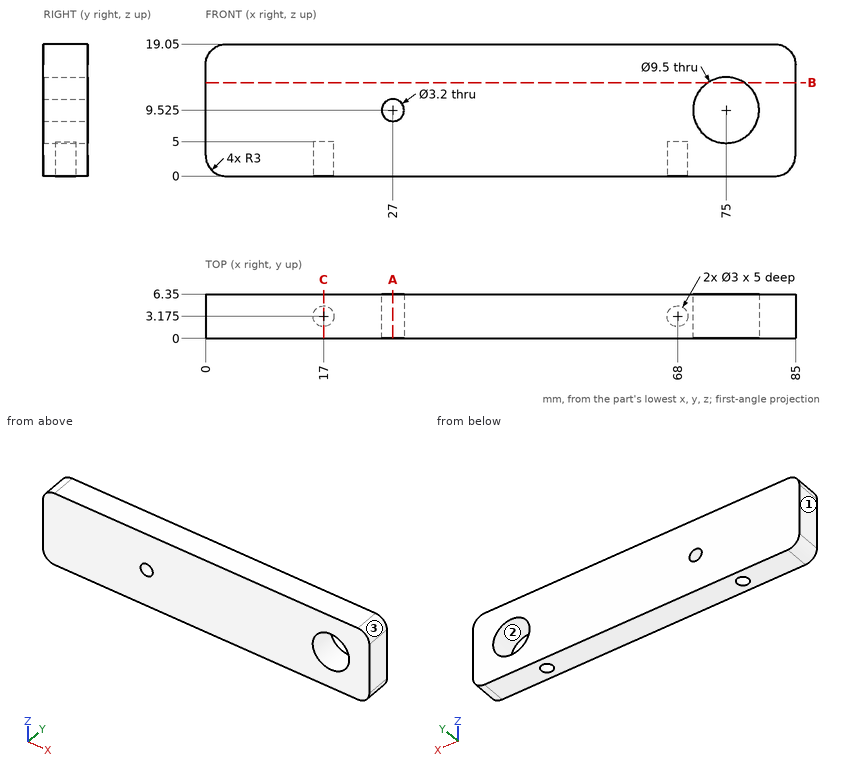
Geometry: see drawing. Coordinates: mm, zero at the bounding-box minimum. Coordinates: 2 decimals unless noted, no trailing zeros. Write each loop counter-clockwise with the first axis right and the second up, starting at its lowest first coordinate (ties: lowest second). Pieces come first, ordered by that corner, then holes. Notation, with made-up numbers: (83, 84.5) - (128, 84.5) arc R28 ccw to (128, 117.5) - close; hole circle Ø7 at (63.5, 61). An arc over 180 degrees is marked (long way). Put each result on its own line as item: value. Start each with the question number.
1) Contact query for flat-ended pins moving along their axis: pin 1 (5.5 mm diameter, centred on x = 75, z = 9.525, fed in from +Y); pin 2 (0.9 mm diameter, centred on x = 17, y = 3.5, fed in from -Z). Output: stop coordinate, or through.
2) Cut plane C-C (x = 17). Return the cut outline in (y, z) (3 decimals), plus the area to 3 significant figures.
3) Cut plane B-B (z = 13.5). Return the cut outline in (x, y).
4) Ray query, L1, parallel to Z at x = 75, y = 3.5 (3 decimals); L2, parallel to X at y = 4.75, z = 10.5; L3, parallel to Z at x = 27, y = 2.75 (3 decimals). Return the intervals inside material, ascending.
5) Cut plane A-A (x = 27). Return the cut outline in (y, z) (3 decimals).
6) Mould query, pull axis X, two halves, no side actions, for the marked faces 1, 2 and 3. Classes: pulls with the +X half, pulls with the -X half, needs draft (parallel to the pull), parting line crosses it, or undercut.
Resolved:
1. pin 1: passes through
1. pin 2: stops at z = 5
2. outline: (0, 0) - (1.675, 0) - (1.675, 5) - (4.675, 5) - (4.675, 0) - (6.35, 0) - (6.35, 19.05) - (0, 19.05) - close
2. area: 106 mm2
3. outline: (0, 0) - (72.4, 0) - (72.4, 6.35) - (0, 6.35) - close; (77.6, 0) - (85, 0) - (85, 6.35) - (77.6, 6.35) - close
4. L1: z = 0 to 4.775, 14.275 to 19.05
4. L2: x = 0 to 25.73, 28.27 to 70.35, 79.65 to 85
4. L3: z = 0 to 7.925, 11.125 to 19.05
5. outline: (0, 0) - (6.35, 0) - (6.35, 7.925) - (0, 7.925) - close; (0, 11.125) - (6.35, 11.125) - (6.35, 19.05) - (0, 19.05) - close
6. face 1: pulls with the -X half
6. face 2: undercut
6. face 3: pulls with the +X half
